from build123d import *

# Parameters (mm, degrees)
SKETCH1_W                         = 43.9928
SKETCH1_H                         = 43.9928
EXTRUDE1_DEPTH                    = 11.43
M2X0_4_TAPPED_HOLE1_AT_2_COUNT    = 2
M2X0_4_TAPPED_HOLE1_AT_2_PITCH    = 34
M2X0_4_TAPPED_HOLE1_AT_3_COUNT    = 2
M2X0_4_TAPPED_HOLE1_AT_3_PITCH    = 48.083261121
M2X0_4_TAPPED_HOLE1_AT_4_COUNT    = 2
M2X0_4_TAPPED_HOLE1_AT_4_PITCH    = 34
FILLET1_R                         = 2.54
FILLET2_R                         = 0.762
FILLET3_R                         = 1.27
SKETCH8_W                         = 43.9928
SKETCH8_H                         = 14.7828
CUT_EXTRUDE1_DEPTH                = 7.112
F_3_8_CLEARANCE_HOLE1_D           = 10.0838
F_3_8_CLEARANCE_HOLE1_CSINK_D     = 11.3538
F_3_8_CLEARANCE_HOLE1_CSINK_ANGLE = 90
CUT_EXTRUDE2_DEPTH                = 4.9964
FILLET4_R                         = 2.54


with BuildPart() as part:
    # Sketch1 → Extrude1 (new body)
    with BuildSketch(Plane(origin=(0, 0, 0), x_dir=(1, 0, 0), z_dir=(0, 1, 0))):
        Rectangle(SKETCH1_W, SKETCH1_H)
    extrude(amount=EXTRUDE1_DEPTH)

    # Sketch2 → M2x0.4 Tapped Hole1 (revolve, cut)
    with BuildSketch(Plane(origin=(-17, 11.43, -17), x_dir=(0, 0, 1), z_dir=(1, 0, 0))):
        Polygon((0, 0), (0, 11.43), (0.8, 11.43), (0.8, 8.001), (1, 8.001), (1, 0.577350269), (2, 0), align=None)
    m2x0_4_tapped_hole1 = revolve(axis=Axis((-17, 17.78, -17), (0, -1, 0)), mode=Mode.SUBTRACT)

    # M2x0.4 Tapped Hole1 at 2: M2x0.4 Tapped Hole1 ×2
    with Locations(*[(0, 0, i * M2X0_4_TAPPED_HOLE1_AT_2_PITCH) for i in range(1, M2X0_4_TAPPED_HOLE1_AT_2_COUNT)]):
        add(m2x0_4_tapped_hole1, mode=Mode.SUBTRACT)

    # M2x0.4 Tapped Hole1 at 3: M2x0.4 Tapped Hole1 ×2
    with Locations(*[Vector(0.707106781, 0, 0.707106781) * (i * M2X0_4_TAPPED_HOLE1_AT_3_PITCH) for i in range(1, M2X0_4_TAPPED_HOLE1_AT_3_COUNT)]):
        add(m2x0_4_tapped_hole1, mode=Mode.SUBTRACT)

    # M2x0.4 Tapped Hole1 at 4: M2x0.4 Tapped Hole1 ×2
    with Locations(*[(i * M2X0_4_TAPPED_HOLE1_AT_4_PITCH, 0, 0) for i in range(1, M2X0_4_TAPPED_HOLE1_AT_4_COUNT)]):
        add(m2x0_4_tapped_hole1, mode=Mode.SUBTRACT)

    # Fillet1
    fillet1_edges = [part.edges().sort_by_distance(p)[0] for p in [
        (-21.9964, 5.715, -21.9964),
        (21.9964, 5.715, -21.9964),
        (21.9964, 5.715, 21.9964),
        (-21.9964, 5.715, 21.9964),
    ]]
    fillet(fillet1_edges, radius=FILLET1_R)

    # Sketch5 → Revolve2 (revolve)
    with BuildSketch(Plane(origin=(0, 0, 0), x_dir=(0, 0, -1), z_dir=(1, 0, 0)), mode=Mode.PRIVATE) as revolve2_sk:
        with BuildLine():
            Line((-20.32, -3.018986953), (-20.32, 0))
            Line((-20.32, 0), (0, 0))
            Line((0, 0), (0, -7.903112155))
            Line((0, -7.903112155), (-8.615503825, -7.903112155))
            ThreePointArc((-8.615503825, -7.903112155), (-14.67240659, -5.951491505), (-20.32, -3.018986953))
        make_face()
    revolve(revolve2_sk.sketch.rotate(Axis((0, -19.634058574, 0), (0, 1, 0)), 180), axis=Axis((0, -19.634058574, 0), (0, 1, 0)))  # turned: the seam where the file's is

    # Fillet2
    fillet2_edges = [part.edges().sort_by_distance(p)[0] for p in [
        (0, 0, 20.32),
    ]]
    fillet(fillet2_edges, radius=FILLET2_R)

    # Fillet3
    fillet3_edges = [part.edges().sort_by_distance(p)[0] for p in [
        (0, -3.018986953, 20.32),
    ]]
    fillet(fillet3_edges, radius=FILLET3_R)

    # Sketch8 → Cut-Extrude1 (cut)
    with BuildSketch(Plane(origin=(0, 11.43, 0), x_dir=(1, 0, 0), z_dir=(0, 1, 0))):
        Rectangle(SKETCH8_W, SKETCH8_H)
    extrude(amount=-CUT_EXTRUDE1_DEPTH, mode=Mode.SUBTRACT)

    # 3/8 Clearance Hole1 (through all)
    with Locations(Plane(origin=(-2.697409808, 4.318, -0.911996033), x_dir=(-1, 0, 0), z_dir=(0, 1, 0))):
        with Locations((-2.697409808, 0.911996033)):
            CounterSinkHole(F_3_8_CLEARANCE_HOLE1_D / 2, F_3_8_CLEARANCE_HOLE1_CSINK_D / 2, counter_sink_angle=F_3_8_CLEARANCE_HOLE1_CSINK_ANGLE)

    # Sketch9 → Cut-Extrude2 (cut)
    with BuildSketch(Plane.ZY.offset(21.9964)):
        Polygon((-17.508, 11.43), (-17, 10.922), (-16.492, 11.43), align=None)
        Polygon((16.492, 11.43), (17, 10.922), (17.508, 11.43), align=None)
    cut_extrude2 = extrude(amount=-CUT_EXTRUDE2_DEPTH, mode=Mode.SUBTRACT)

    # Mirror1: Cut-Extrude2 across plane
    add(cut_extrude2.mirror(Plane(origin=(0, 0, 0), x_dir=(0, 0, 1), z_dir=(1, 0, 0))), mode=Mode.SUBTRACT)

    # Fillet4
    fillet4_edges = [part.edges().sort_by_distance(p)[0] for p in [
        (0, -7.903112155, 8.615503825),
    ]]
    fillet(fillet4_edges, radius=FILLET4_R)


solid = part.part
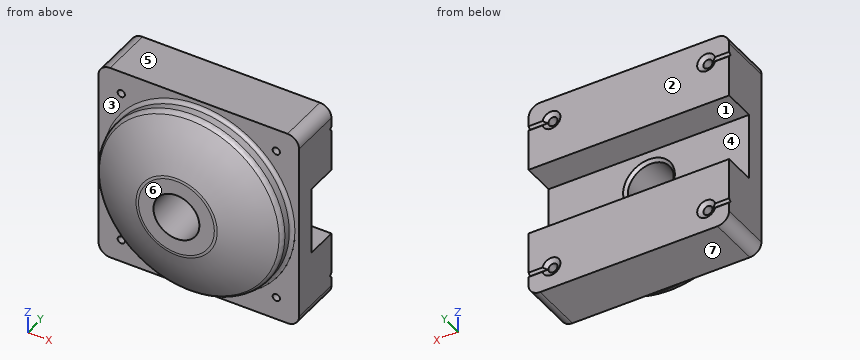
Geometry: final body of the model. Coordinates: model frame, mm. Face numbers are marked on the shaded views. A direction names the side the tool comes from. Coordinates: 2 decimals unless noted, no trailing zeros. Loops run counter-clockwise (first coordinate to the right, second up) from the corner with the lowest first, then second, coordinate; pieces in that order, holes last. Notation, with made-up numbers: M 44.25,-9 L 75.25,-9 A14 cw 75.25,9 Z; hole C 86,-27.5 d7. An arc over 180 degrees is marked long. One line per item, written item: value. Start each with the question number.
1) Material intervals for L1, parallel to Z at x = -17, y = 9.5; L2, parallel to X at y = 0.7, z = 17, sorted ascending. Write a range as from..to.
2) Cut plane A-A (y = 9.5). Return loops of the section in (x, z).
3) Cut plane D-D (y = -6.5). Return loops of the section in (x, z).
4) Cut plane B-B (y = 2.25). Return loops of the section in (x, z), then the cut area to 3 significant figures.
5) Pin query (flat end, axial travel): P1, Ø2.5, axis at x = 17, z = -17, coming from the +Y side; P2, Ø10, axis at x = 5, z = -12, coming from the -Y side; P3, Ø12, axis at x = 15, z = -4, coming from the -Y side; P4, Ø5, axis at x = -11.5, z = -16.5, coming from the -Y side. Return the tip coordinate at first contact, or that it passes through.
6) Reachability of the marked faces 1, 2 and 3 from +Z, -Z, +X, -X, +Y, -Y: full face, straight path, thin tool, end or side. Return the list, or none.
7) Draft query along Z for the marked faces 4, 5, 6 and 7. Return one class per face: released by +Z, released by -Z, zero draft, split by the parting line, or undercut.
8) Cut plane C-C (x = -17). Count the separate pieces of the cut face and the enclosed holes in it, then the cut area to 3 significant figures.
Evaluation:
1. L1: -22..-18, -16..-7.39, 7.39..16, 18..22
1. L2: -22..-17.8, -16.2..16.2, 17.8..22
2. outline: M -22,-19.46 A2.54 ccw -19.46,-22 L 19.46,-22 A2.54 ccw 22,-19.46 L 22,-7.39 L -22,-7.39 Z; M -22,7.39 L 22,7.39 L 22,19.46 A2.54 ccw 19.46,22 L -19.46,22 A2.54 ccw -22,19.46 Z; hole C -17,-17 d2; hole C -17,17 d2; hole C 17,-17 d2; hole C 17,17 d2
3. outline: C 0,0 d26.56; hole C 0,0 d10.08
4. outline: M -22,-19.46 A2.54 ccw -19.46,-22 L 19.46,-22 A2.54 ccw 22,-19.46 L 22,19.46 A2.54 ccw 19.46,22 L -19.46,22 A2.54 ccw -22,19.46 Z; hole C -17,-17 d1.6; hole C -17,17 d1.6; hole C 0,0 d10.08; hole C 17,-17 d1.6; hole C 17,17 d1.6
4. area: 1,840 mm^2
5. P1: y = 11
5. P2: y = -7.9
5. P3: y = -7.68
5. P4: y = -4.57
6. face 1: +X, -X, +Y
6. face 2: +Z, -Z, +X, -X, +Y
6. face 3: -Y
7. face 4: undercut
7. face 5: released by +Z
7. face 6: zero draft
7. face 7: released by -Z
8. separate pieces: 3
8. enclosed holes: 0
8. area: 449 mm^2
